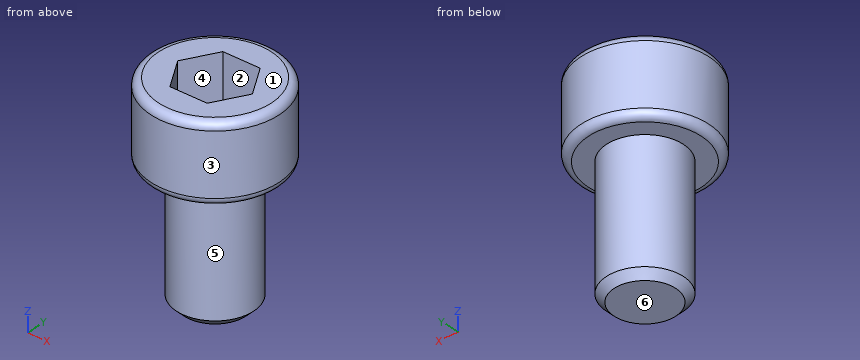
from build123d import *

# Parameters (mm, degrees)
SKETCH_1_R          = 2.5
EXTRUDE_1_DEPTH     = 3
SKETCH_2_R          = 1.5
EXTRUDE_2_DEPTH     = 5
CUT_EXTRUDE_1_DEPTH = 2
CHAMFER_1_SIZE      = 0.3
FILLET_1_R          = 0.3


with BuildPart() as part:
    # 草图1 → 凸台-拉伸1 (new body)
    with BuildSketch(Plane.XY):
        Circle(SKETCH_1_R)
    extrude(amount=EXTRUDE_1_DEPTH)

    # 草图2 → 凸台-拉伸2 (add)
    with BuildSketch(Plane(origin=(0, 0, 0), x_dir=(-1, 0, 0), z_dir=(0, 0, -1))):
        Circle(SKETCH_2_R)
    extrude(amount=EXTRUDE_2_DEPTH)

    # 草图3 → 切除-拉伸1 (cut)
    with BuildSketch(Plane.XY.offset(3)):
        Polygon((1.443375673, 0), (0.721687836, 1.25), (-0.721687836, 1.25), (-1.443375673, 0), (-0.721687836, -1.25), (0.721687836, -1.25), align=None)
    extrude(amount=-CUT_EXTRUDE_1_DEPTH, mode=Mode.SUBTRACT)

    # 倒角1
    chamfer_1_edges = [part.edges().sort_by_distance(p)[0] for p in [
        (1.5, 0, -5),
    ]]
    chamfer(chamfer_1_edges, length=CHAMFER_1_SIZE)

    # 圆角1
    fillet_1_edges = [part.edges().sort_by_distance(p)[0] for p in [
        (-2.5, 0, 0),
        (-2.5, 0, 3),
    ]]
    fillet(fillet_1_edges, radius=FILLET_1_R)


solid = part.part
Design review of the part built by this model. Coordinates are the model's own, in mm. Face numbers are marked on the shaded views. A direction names the side the tool comes from. Give positions to 0.01 mm unless a question says otherwise; leave off trailing zeros. Order: outer loops, then holes, each group sorted by start corner. A loop starts at its lowest first (then second) coordinate and runs counter-clockwise, first axis right, second up. Notation, with made-up numbers: (-18.5, 86.25) - (34.5, 86.25) arc R5 ccw to (34.5, 93.25) - close; hole circle Ø7 at (66.5, 23.5). An arc over 180 degrees is marked (long way). Use CSV: the item, a comma, the result in double quotes. Start each with the question number.
Q1. For P1, Ø1.5, axis at x = 1.5, z = 0.5, coming from the +Y side; P2, Ø2, axis at y = -1.5, z = -0.5, coming from the +X side; P3, Ø2, axis at x = -1.5, z = 2, coming from the -Y side, all flat-tipped, find the tip position at first contact; note any pin that passes through.
Q2. Machinability: for the marked faces 4, 5 and 6, which of the approach directions +Z, -Z, +X, -X, +Y, -Y give a long, thin tool a straight path to every point of the face, cutting with its end or side? Answer none if there is none.
Q3. Draft analysis for pull direction Y (two halves, no side actions). For the marked faces 1, 2 and 3, state which applies: pulls with the +Y half, pulls with the -Y half, needs draft (parallel to the pull), parting line crosses it, or undercut.
Q4. For line 1 (Z direction, x = 0.85, y = 0.65); line 2 (X direction, y = -2, z = 1.25); line 3 (Z direction, x = 0.8, y = 1.4), list the stretches that pass through material, from the lowest coordinate up.
Q5. Take a section at B-B (z = -3.25). State the section outline as (x, y) points, and give its area (3 significant figures).
Q6. Take a section at A-A (x = 0). State the section outline as (y, z) points, and give its area (3 significant figures).
Calculated:
1,P1,"stops at y = 2.38"
1,P2,"stops at x = 2.36"
1,P3,"stops at y = -2.45"
2,face 4,"+Z"
2,face 5,"-Z"
2,face 6,"-Z, +X, -X, +Y, -Y"
3,face 1,"needs draft"
3,face 2,"undercut"
3,face 3,"parting line crosses it"
4,line 1,"z = -5 to 1"
4,line 2,"x = -1.5 to 1.5"
4,line 3,"z = 0 to 3"
5,outline,"circle Ø3 at (0, 0)"
5,area,"7.07 mm²"
6,outline,"(-2.5, 0.3) arc R0.3 ccw to (-2.2, 0) - (-1.5, 0) - (-1.5, -4.7) - (-1.2, -5) - (1.2, -5) - (1.5, -4.7) - (1.5, 0) - (2.2, 0) arc R0.3 ccw to (2.5, 0.3) - (2.5, 2.7) arc R0.3 ccw to (2.2, 3) - (1.25, 3) - (1.25, 1) - (-1.25, 1) - (-1.25, 3) - (-2.2, 3) arc R0.3 ccw to (-2.5, 2.7) - close"
6,area,"24.8 mm²"
